from build123d import *

# Parameters (mm, degrees)
F1_DEPTH = 7.9375


with BuildPart() as f1:
    # F0 (on Right) → F1 (new body)
    with BuildSketch(Plane.YZ):
        with BuildLine():
            ThreePointArc((-45.24375, 0), (0, 45.24375), (45.24375, 0))
            Line((45.24375, 0), (93.1603, 43.353069))
            ThreePointArc((93.1603, 43.353069), (94.704111, 45.486011), (95.25, 48.061821))
            Line((95.25, 48.061821), (95.25, 76.99375))
            ThreePointArc((95.25, 76.99375), (93.390128, 81.483878), (88.9, 83.34375))
            Line((88.9, 83.34375), (57.15, 83.34375))
            Line((57.15, 83.34375), (57.15, 89.69375))
            Line((57.15, 89.69375), (38.1, 89.69375))
            Line((38.1, 89.69375), (38.1, 83.34375))
            Line((38.1, 83.34375), (-38.1, 83.34375))
            Line((-38.1, 83.34375), (-38.1, 89.69375))
            Line((-38.1, 89.69375), (-57.15, 89.69375))
            Line((-57.15, 89.69375), (-57.15, 83.34375))
            Line((-57.15, 83.34375), (-88.9, 83.34375))
            ThreePointArc((-88.9, 83.34375), (-93.390128, 81.483878), (-95.25, 76.99375))
            Line((-95.25, 76.99375), (-95.25, 48.061821))
            ThreePointArc((-95.25, 48.061821), (-94.704111, 45.486011), (-93.1603, 43.353069))
            Line((-93.1603, 43.353069), (-45.24375, 0))
        make_face()
    extrude(amount=F1_DEPTH)


solid = f1.part
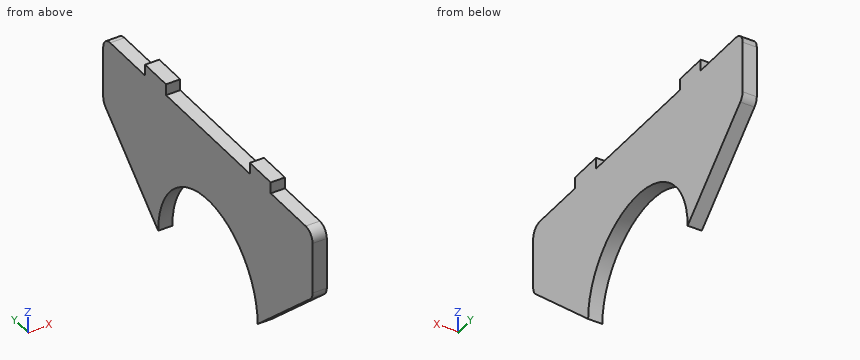
Could you check a few things on this model? Use its own coordinates, in mm. Round coordinates to 2 decimals unless told otherwise and drop trailing zeros. Write each loop counter-clockwise with the first axis right and the second up, starting at its lowest first coordinate (ties: lowest second). Pieces come first, ordered by that corner, then holes. Notation, with made-up numbers: (35, 77.25) - (55, 77.25) arc R33 cw to (55, 108.25) - close; hole circle Ø10 at (72, 28.25). An arc over 180 degrees is marked (long way). Use a Markdown table: item, result.
Q1. I want a section at C-C (y = 0). List the corners of the cut face in (x, z) for me.
Output values:
| item | result |
|---|---|
| outline | (0, 45.24) - (7.94, 45.24) - (7.94, 83.34) - (0, 83.34) - close |
Q2. Please list where these lines run through material, in increasing order: L1, parallel to Y at x = 1, z = 31; L2, parallel to Z at x = 5.25, y = 0.5; L3, parallel to Y at x = 3, z = 17.
Output values:
| item | result |
|---|---|
| L1 | -79.51 to -32.95, 32.95 to 79.51 |
| L2 | 45.24 to 83.34 |
| L3 | -64.03 to -41.93, 41.93 to 64.03 |
Q3. For pin 1 (1 mm diameter, centred on x = 2.5, y = 8.5, fed in from -Z); pin 2 (1.9 mm diameter, centred on x = 4, z = 86, fed in from +Y); pin 3 (2.5 mm diameter, centred on x = 2.5, y = 75.5, fed in from +Z), each with a flat end and sliding along its axis, tell me the tip position at first contact or that it passes through.
Output values:
| item | result |
|---|---|
| pin 1 | z = 44.34 |
| pin 2 | y = 57.15 |
| pin 3 | z = 83.34 |
Q4. I want a section at D-D (z = 12). List the corners of the cut face in (x, y) for me.
Output values:
| item | result |
|---|---|
| outline | (0, -58.51) - (7.94, -58.51) - (7.94, -43.62) - (0, -43.62) - close; (0, 43.62) - (7.94, 43.62) - (7.94, 58.51) - (0, 58.51) - close |
Q5. I want a section at A-A (z = 34.5). List the corners of the cut face in (x, y) for me.
Output values:
| item | result |
|---|---|
| outline | (0, -83.38) - (7.94, -83.38) - (7.94, -29.27) - (0, -29.27) - close; (0, 29.27) - (7.94, 29.27) - (7.94, 83.38) - (0, 83.38) - close |
Q6. I want a section at B-B (x = 4.25). List the corners of the cut face in (y, z) for me.
Output values:
| item | result |
|---|---|
| outline | (-95.25, 48.06) arc R6.35 ccw to (-93.16, 43.35) - (-45.24, 0) arc R45.24 cw to (45.24, 0) - (93.16, 43.35) arc R6.35 ccw to (95.25, 48.06) - (95.25, 76.99) arc R6.35 ccw to (88.9, 83.34) - (57.15, 83.34) - (57.15, 89.69) - (38.1, 89.69) - (38.1, 83.34) - (-38.1, 83.34) - (-38.1, 89.69) - (-57.15, 89.69) - (-57.15, 83.34) - (-88.9, 83.34) arc R6.35 ccw to (-95.25, 76.99) - close |
